Design review of the part built by this model. Coordinates are the model's own, in mm. Round coordinates to 2 decimals unless told otherwise and drop trailing zeros. Order: outer loops, then holes, each group sorted by start corner. A loop starts at its lowest first (then second) coordinate and runs counter-clockwise, first axis right, second up. Notation, with made-up numbers: (8, -6.5) - (51, -6.5) arc R5 cw to (51, -1.5) - close; hole circle Ø2 at (6.5, -26.75). An arc over 180 degrees is marked (long way). Answer as a JSON object with one key per item and string values. Group by question number.
from build123d import *

# Parameters (mm, degrees)
EXTRUDE_1_DEPTH        = 12
SKETCH_2_W             = 40
SKETCH_2_H             = 6
CUT_EXTRUDE_1_DEPTH    = 6.5
DRAFT_1_ANGLE          = 45
DRAFT_2_ANGLE          = 45
PATTERN_START          = 4
PATTERN_LINEAR_1_DEPTH = 6
MIRROR_START           = 4
MIRROR_2_DEPTH         = 6
CUT_EXTRUDE_START      = -2
CUT_EXTRUDE_2_DEPTH    = 6


# Read off the part's stored shape, not the designer's step: 阵列(线性)1, 镜向2
with BuildPart() as part:
    # 草图1 → 凸台-拉伸1 (new body)
    with BuildSketch(Plane.XY):
        Polygon((0, 12), (0, 5), (27, 5), (27, -5), (0, -5), (0, -12), (862, -12), (886, 12), align=None)
    extrude(amount=EXTRUDE_1_DEPTH)

    # 草图2 → 切除-拉伸1 (cut)
    with BuildSketch(Plane.XZ.offset(12)):
        with Locations((175, 7)):
            Rectangle(SKETCH_2_W, SKETCH_2_H)
    extrude(amount=-CUT_EXTRUDE_1_DEPTH, mode=Mode.SUBTRACT)

    # 拔模1
    draft_1_faces = [part.faces().sort_by_distance(p)[0] for p in [
        (155, -8.75, 7),
    ]]
    draft(draft_1_faces, Plane(origin=(0, -5.5, 0), x_dir=(0, 0, -1), z_dir=(0, -1, 0)), DRAFT_1_ANGLE)

    # 拔模2
    draft_2_faces = [part.faces().sort_by_distance(p)[0] for p in [
        (195, -8.75, 7),
    ]]
    draft(draft_2_faces, Plane(origin=(0, -5.5, 0), x_dir=(0, 0, -1), z_dir=(0, -1, 0)), DRAFT_2_ANGLE)

    # 阵列(线性)1 outline → 阵列(线性)1 (cut)
    with BuildSketch(Plane.XY.offset(PATTERN_START)):
        Polygon((551.5, -12), (545, -5.5), (505, -5.5), (498.5, -12), align=None)
    extrude(amount=PATTERN_LINEAR_1_DEPTH, mode=Mode.SUBTRACT)

    # 镜向2 outline → 镜向2 (cut)
    with BuildSketch(Plane.XY.offset(MIRROR_START)):
        Polygon((195, 5.5), (201.5, 12), (148.5, 12), (155, 5.5), align=None)
        Polygon((545, 5.5), (551.5, 12), (498.5, 12), (505, 5.5), align=None)
    extrude(amount=MIRROR_2_DEPTH, mode=Mode.SUBTRACT)

    # 草图4 → 切除-拉伸2 (cut)
    with BuildSketch(Plane.XY.offset(12).offset(CUT_EXTRUDE_START)):
        Polygon((832.5, 12), (839, 5.5), (879.5, 5.5), (886, 12), align=None)
        Polygon((832.5, -12), (839, -5.5), (868.5, -5.5), (862, -12), align=None)
    extrude(amount=-CUT_EXTRUDE_2_DEPTH, mode=Mode.SUBTRACT)


solid = part.part
1. To check wall thickness, follow line 1 (X direction, y = 10.25, z = 6.25); line 2 (X direction, y = -8.5, z = 6.5); line 3 (Y direction, x = 177, z = 8.5). State the ranges of each line that lie inside material, in increasing order. Write a range as from..to.
2. Take a section at B-B, the plane z = 7. Give the boundary of the cut face in (x, y).
3. Take a section at A-A, the plane x = 520. Give the boundary of the cut face in (y, z).
4. Take a section at C-C, the plane y = -0.5. Give the boundary of the cut face in (x, z), then the cut area to 3 significant figures.
5. Clearance check with flat-ended pins moving along their axes: P1, Ø12, axis at x = 548, y = -1, coming from the -Z side; P2, Ø4, axis at y = 0.5, z = 4, coming from the +X side; P3, Ø1.8, axis at x = 862, z = 5.5, coming from the +Y side; P4, Ø3, axis at y = -1, z = 6, coming from the -X side. State where each tip first meets the part, or that it passes through.
Response values:
{
 "1": {"line 1": "0..150.25, 199.75..500.25, 549.75..834.25", "line 2": "0..152, 198..502, 548..836", "line 3": "-5.5..5.5"},
 "2": {"outline": "(0, -12) - (148.5, -12) - (155, -5.5) - (195, -5.5) - (201.5, -12) - (498.5, -12) - (505, -5.5) - (545, -5.5) - (551.5, -12) - (832.5, -12) - (839, -5.5) - (868.5, -5.5) - (879.5, 5.5) - (839, 5.5) - (832.5, 12) - (551.5, 12) - (545, 5.5) - (505, 5.5) - (498.5, 12) - (201.5, 12) - (195, 5.5) - (155, 5.5) - (148.5, 12) - (0, 12) - (0, 5) - (27, 5) - (27, -5) - (0, -5) - close"},
 "3": {"outline": "(-12, 0) - (12, 0) - (12, 4) - (5.5, 4) - (5.5, 10) - (12, 10) - (12, 12) - (-12, 12) - (-12, 10) - (-5.5, 10) - (-5.5, 4) - (-12, 4) - close"},
 "4": {"outline": "(27, 0) - (873.5, 0) - (873.5, 12) - (27, 12) - close", "area": "10,200 mm2"},
 "5": {"P1": "z = 0", "P2": "x = 876.5", "P3": "y = 5.5", "P4": "x = 27"}
}
